from build123d import *

# Parameters (mm, degrees)
F0_R     = 16.05
F1_DEPTH = 2.7
F2_R     = 16.05
F2_R_2   = 15.05
F3_DEPTH = 2
F4_R     = 0.99999
F5_R     = 16.05
F6_DEPTH = 0.5


# Not quite as in the source:
# - a fillet or chamfer is up to 0.001 mm smaller than in the source, because OpenCascade refuses the exact size


with BuildPart() as f1:
    # F0 (on Top) → F1 (new body)
    with BuildSketch(Plane.XY):
        Circle(F0_R)
        with BuildLine():
            ThreePointArc((-0.6780739779, -9.7725818409), (-1.4027582732, -9.0367076796), (-1.7421252674, -8.061254886))
            ThreePointArc((-1.7421252674, -8.061254886), (-4.3074337596, -3.0577956653), (-9.536973063, -0.9920438631))
            ThreePointArc((-9.536973063, -0.9920438631), (-11.3022646183, -0.0029612607), (-11.6691612698, 1.9869948988))
            Line((-11.6691612698, 1.9869948988), (-9.4391799782, 10.4875703743))
            ThreePointArc((-9.4391799782, 10.4875703743), (-9.0171024282, 11.1985139757), (-8.2824484024, 11.5778208766))
            Line((-8.2824484024, 11.5778208766), (-6.0604061806, 12.0222295772))
            ThreePointArc((-6.0604061806, 12.0222295772), (-5.5105978167, 12.029415178), (-4.9951399441, 11.8379888177))
            Line((-4.9951399441, 11.8379888177), (4.893855989, 5.9114030387))
            ThreePointArc((4.893855989, 5.9114030387), (5.3199805506, 5.5689093688), (5.6374422976, 5.1238227536))
            Line((5.6374422976, 5.1238227536), (12.1259901628, -7.2648903372))
            ThreePointArc((12.1259901628, -7.2648903372), (12.1554437407, -8.5973863607), (11.1125476049, -9.4273145597))
            Line((11.1125476049, -9.4273145597), (2.1831787086, -11.347409045))
            ThreePointArc((2.1831787086, -11.347409045), (1.5325569034, -11.3429782119), (0.9450171886, -11.0634689113))
            Line((0.9450171886, -11.0634689113), (-0.6780739779, -9.7725818409))
        make_face(mode=Mode.SUBTRACT)
    extrude(amount=F1_DEPTH)

    # F2 (on face) → F3 (join)
    with BuildSketch(Plane.XY.offset(2.7)):
        Circle(F2_R)
        Circle(F2_R_2, mode=Mode.SUBTRACT)
    extrude(amount=F3_DEPTH)

    # F4 (radius 1 in the source; OpenCascade refuses exactly that, so slightly less here)
    f4_edges = [f1.edges().sort_by_distance(p)[0] for p in [
        (-16.05, 0, 4.7),
    ]]
    fillet(f4_edges, radius=F4_R)

    # F5 (on face) → F6 (join)
    with BuildSketch(Plane.XY):
        Circle(F5_R)
    extrude(amount=F6_DEPTH)


solid = f1.part
Source: CAD feature listing. Evaluate the final solid. Frame: model axes, mm. Give positions to 0.01 mm unless a question says otherwise; leave off trailing zeros. Loops run counter-clockwise (first coordinate to the right, second up) from the corner with the lowest first, then second, coordinate; pieces in that order, holes last. Notation, with made-up numbers: (-31.5, 78) -> (10.5, 78) arc R25 cw to (10.5, 113) -> close; hole circle Ø8 at (21.25, 78.25). An arc over 180 degrees is marked (long way). Use a Markdown table: item, result. Add a question column.
1) Section query A-A, the plane z = 2.3. Return the cut outline in (x, y), then the cut area to 3 significant figures.
2) Line query: line 1 along Y through (x, z) = (0, 3.5); line 2 along Y through (x, z) = (2.5, 3.8); line 3 along Z through (x, y) = (-7, -2.5). Output: solid intervals per line, ascending. Write a range as [from, to].
3) First-contact query: pin 1 (15 mm diameter, centred on x = -1, y = 1.5, fed in from +Z); pin 2 (10 mm diameter, centred on x = 0, y = -3, fed in from -Z); pin 3 (1 mm diameter, centred on x = 5.5, z = 4, fed in from +Y); pin 4 (1.5 mm diameter, centred on x = -3, z = 1.5, fed in from +Y). Flat tips, straight axial feed; report the tip coordinate or a pass-through.
4) Pull-direction query (Y, two-part tool) for faces 1 (the face through (0, 0, 0)), 2 (the face through (-1.395, -9.049, 1.585)), 3 (the face through (-12.737, -9.766, 1.824)); classes: +Y half, -Y half, draft (parallel to the pull), parting line (faces both ways), or undercut.
Numbers:
| question | item | result |
|---|---|---|
| 1 | outline | circle Ø32.1 at (0, 0); hole (-11.67, 1.99) arc R2.38 ccw to (-9.54, -0.99) arc R7.97 cw to (-1.74, -8.06) arc R2.35 ccw to (-0.68, -9.77) -> (0.95, -11.06) arc R1.5 ccw to (2.18, -11.35) -> (11.11, -9.43) arc R1.5 ccw to (12.13, -7.26) -> (5.64, 5.12) arc R2 ccw to (4.89, 5.91) -> (-5, 11.84) arc R1.5 ccw to (-6.06, 12.02) -> (-8.28, 11.58) arc R1.5 ccw to (-9.44, 10.49) -> close |
| 1 | area | 493 mm2 |
| 2 | line 1 | y = [-16.05, -15.05], [15.05, 16.05] |
| 2 | line 2 | y = [-15.85, -14.84], [14.84, 15.85] |
| 2 | line 3 | z = [0, 2.7] |
| 3 | pin 1 | stops at z = 2.7 |
| 3 | pin 2 | stops at z = 0 |
| 3 | pin 3 | stops at y = 15.23 |
| 3 | pin 4 | stops at y = 15.89 |
| 4 | face 1 | draft |
| 4 | face 2 | undercut |
| 4 | face 3 | parting line |
